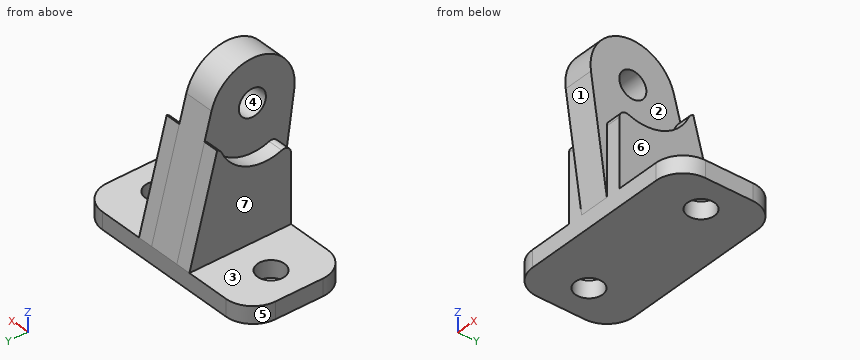
```python
from build123d import *

# Parameters (mm, degrees)
SZKIC1_R                         = 4
DODANIE_WYCI_GNI_CIE1_DEPTH      = 5
SZKIC7_R                         = 4
DODANIE_WYCI_GNI_CIE3_DEPTH      = 4.5
DODANIE_WYCI_GNI_CIE5_DEPTH      = 4.5
DODANIE_WYCI_GNI_CIE5_DEPTH_BACK = 13.5


with BuildPart() as part:
    # Szkic1 → Dodanie-wyciągnięcie1 (new body)
    with BuildSketch(Plane.XY):
        with BuildLine():
            Line((-22, 15), (22, 15))
            ThreePointArc((22, 15), (27.656854249, 12.656854249), (30, 7))
            Line((30, 7), (30, -7))
            ThreePointArc((30, -7), (27.656854249, -12.656854249), (22, -15))
            Line((22, -15), (-22, -15))
            ThreePointArc((-22, -15), (-27.656854249, -12.656854249), (-30, -7))
            Line((-30, -7), (-30, 7))
            ThreePointArc((-30, 7), (-27.656854249, 12.656854249), (-22, 15))
        make_face()
        with Locations((-20, 0)):
            Circle(SZKIC1_R, mode=Mode.SUBTRACT)
        with Locations((20, 0)):
            Circle(SZKIC1_R, mode=Mode.SUBTRACT)
    extrude(amount=DODANIE_WYCI_GNI_CIE1_DEPTH)

    # Szkic7 → Dodanie-wyciągnięcie3 (add, symmetric)
    with BuildSketch(Plane(origin=(0, 0, 0), x_dir=(0, 0, -1), z_dir=(1, 0, 0))):
        with BuildLine():
            Line((-5, 15), (-43.235238064, 4.754898838))
            ThreePointArc((-43.235238064, 4.754898838), (-52.248209815, -9.815442471), (-38.251909732, -19.696337656))
            Line((-38.251909732, -19.696337656), (-5, -15))
            Line((-5, -15), (-5, 15))
        make_face()
        with Locations((-40, -7.31917399)):
            Circle(SZKIC7_R, mode=Mode.SUBTRACT)
    extrude(amount=DODANIE_WYCI_GNI_CIE3_DEPTH, both=True)

    # Szkic8 → Dodanie-wyciągnięcie5 (add, two sides: drawn at the far end of the back side and taken through both)
    with BuildSketch(Plane(origin=(4.5, 0, 0), x_dir=(0, 0, -1), z_dir=(1, 0, 0)).offset(-DODANIE_WYCI_GNI_CIE5_DEPTH_BACK)):
        with BuildLine():
            Line((-5, -15), (-5, 15))
            Line((-5, 15), (-35.519913082, 6.822213937))
            ThreePointArc((-35.519913082, 6.822213937), (-35.104612696, 6.035983837), (-34.389553751, 5.507473775))
            ThreePointArc((-34.389553751, 5.507473775), (-27.092900988, -1.896370741), (-26.91214627, -12.289896749))
            ThreePointArc((-26.91214627, -12.289896749), (-26.688692003, -14.135736214), (-25.04245288, -15))
            Line((-25.04245288, -15), (-5, -15))
        make_face()
    extrude(amount=DODANIE_WYCI_GNI_CIE5_DEPTH + DODANIE_WYCI_GNI_CIE5_DEPTH_BACK)


solid = part.part
```
Geometry check sheet. Reference: the model listing, model coordinates, mm. Face numbers are marked on the shaded views. A direction names the side the tool comes from. Coordinates: 2 decimals unless noted, no trailing zeros. Order: outer loops, then holes, each group sorted by start corner. A loop starts at its lowest first (then second) coordinate and runs counter-clockwise, first axis right, second up.
Q1. Sectioned sample at D-D on z = 31. Record the cut outline in (x, y).
Reply:
outline: (-9, 3.4) - (-4.5, 3.4) - (-4.5, -18.67) - (4.5, -18.67) - (4.5, 3.4) - (9, 3.4) - (9, 8.03) - (-9, 8.03) - close
Q2. Depth check by flat-ended pin: pin 1 Ø6 at (x, y) = (-9.5, -2) entering from +Z; pin 2 Ø8 at (x, y) = (-12.5, -11.5) entering from +Z; pin 3 Ø10.5 at (x, y) = (-18, -4.5) entering from +Z. Enter the tip coordinate at first touch or a pass-through.
Reply:
pin 1: stops at z = 28.71
pin 2: stops at z = 27.04
pin 3: stops at z = 5
Q3. Sectioned sample at C-C on z = 40. Record the cut outline in (x, y), and give its area (3 significant figures).
Reply:
outline: (-4.5, -19.82) - (4.5, -19.82) - (4.5, -11.32) - (-4.5, -11.32) - close; (-4.5, -3.32) - (4.5, -3.32) - (4.5, 5.62) - (-4.5, 5.62) - close
area: 157 mm2
Q4. Thickness scan on probe 1 along Y at (x, z) = (-20, 2.6); probe 2 along X at (y, z) = (10.5, 19); probe 3 along X at (y, z) = (-12.5, 40). Record the ranges inside material, lowest first.
Reply:
probe 1: y = -15 to -4, 4 to 15
probe 2: x = -9 to 9
probe 3: x = -4.5 to 4.5
Q5. Tool access check on the marked faces 5, 6 and 7. Record the directions out of +Z, -Z, +X, -X, +Y, -Y that give a thin tool (end or side, any length) a straight path to the whole face; none if there is none.
Reply:
face 5: +Z, -Z, -X, +Y
face 6: +Z, +X, +Y, -Y
face 7: +Z, -X, +Y, -Y
Q6. Draft check along Z on the marked faces 1, 2, 3 and 4. Enter one of: released by +Z, released by -Z, zero draft, split by the parting line, or undercut.
Reply:
face 1: released by -Z
face 2: zero draft
face 3: released by +Z
face 4: undercut
Q7. Sectioned sample at B-B on x = 20. Record the cut outline in (y, z), and give its area (3 significant figures).
Reply:
outline: (-15, 0) - (-4, 0) - (-4, 5) - (-15, 5) - close; (4, 0) - (15, 0) - (15, 5) - (4, 5) - close
area: 110 mm2
Q8. Sectioned sample at A-A on y = -1. Record the cut outline in (x, z).
Reply:
outline: (-30, 0) - (-23.87, 0) - (-23.87, 5) - (-30, 5) - close; (-16.13, 0) - (16.13, 0) - (16.13, 5) - (9, 5) - (9, 27.51) - (4.5, 27.51) - (4.5, 50.79) - (-4.5, 50.79) - (-4.5, 27.51) - (-9, 27.51) - (-9, 5) - (-16.13, 5) - close; (23.87, 0) - (30, 0) - (30, 5) - (23.87, 5) - close
